Build history of the part. All positions in model axes, mm. A direction names the side the tool comes from. Round coordinates to 2 decimals unless told otherwise and drop trailing zeros. Use one line per item in the form item = value. Start each with the question number.
```python
from build123d import *

# Parameters (mm, degrees)
F0_R     = 37
F1_DEPTH = 2
F2_R     = 38
F3_DEPTH = 3
F4_R     = 37
F5_DEPTH = 2
F6_R     = 38
F7_DEPTH = 3
F8_R     = 37
F9_DEPTH = 2


# Not quite as in the source:
# - a fillet or chamfer that OpenCascade refuses, or shapes differently, is made with other operations: its cross-section is extruded or revolved along the edge and cut away or added


with BuildPart() as f1:
    # F0 (on Top) → F1 (new body)
    with BuildSketch(Plane.XY):
        Circle(F0_R)
    extrude(amount=F1_DEPTH)

    # F2 (on face) → F3 (join)
    with BuildSketch(Plane.XY.offset(2)):
        Circle(F2_R)
    extrude(amount=F3_DEPTH)

    # F4 (on face) → F5 (join)
    with BuildSketch(Plane.XY.offset(5)):
        Circle(F4_R)
    extrude(amount=F5_DEPTH)

    # F6 (on face) → F7 (join)
    with BuildSketch(Plane.XY.offset(7)):
        Circle(F6_R)
    extrude(amount=F7_DEPTH)

    # F8 (on face) → F9 (join)
    with BuildSketch(Plane.XY.offset(10)):
        Circle(F8_R)
    extrude(amount=F9_DEPTH)

    # F10: fillet of radius 1.6 on 4 edges, made by hand

    # F10_s1 → F10_t2 (revolve, cut)
    with BuildSketch(Plane.XZ):
        with BuildLine():
            ThreePointArc((38, 8.4832396974), (37.7266499161, 7.5888125064), (37, 7))
            Line((37, 7), (38, 7))
            Line((38, 7), (38, 8.4832396974))
        make_face()
    revolve(axis=Axis((0, 0, 7), (0, 0, 1)), mode=Mode.SUBTRACT)

    # F10_s3 → F10_t4 (revolve, cut)
    with BuildSketch(Plane.XZ):
        with BuildLine():
            ThreePointArc((38, 3.4832396974), (37.7266499161, 2.5888125064), (37, 2))
            Line((37, 2), (38, 2))
            Line((38, 2), (38, 3.4832396974))
        make_face()
    revolve(axis=Axis((0, 0, 2), (0, 0, 1)), mode=Mode.SUBTRACT)

    # F10_s5 → F10_t6 (revolve, cut)
    with BuildSketch(Plane.XZ):
        with BuildLine():
            ThreePointArc((38, 8.5167603026), (37.7266499161, 9.4111874936), (37, 10))
            Line((37, 10), (38, 10))
            Line((38, 10), (38, 8.5167603026))
        make_face()
    revolve(axis=Axis((0, 0, 10), (0, 0, 1)), mode=Mode.SUBTRACT)

    # F10_s7 → F10_t8 (revolve, cut)
    with BuildSketch(Plane.XZ):
        with BuildLine():
            ThreePointArc((37, 5), (37.7266499161, 4.4111874936), (38, 3.5167603026))
            Line((38, 3.5167603026), (38, 5))
            Line((38, 5), (37, 5))
        make_face()
    revolve(axis=Axis((0, 0, 5), (0, 0, 1)), mode=Mode.SUBTRACT)


solid = f1.part
```
Q1. Drop flat-ended pins along their axis: P1, Ø10, axis at x = 23, y = -30, coming from the +Z side; P2, Ø2, axis at x = -25.5, z = 9, coming from the -Y side; P3, Ø4, axis at y = 9, z = 7.5, coming from the +X side; P4, Ø1.5, axis at y = -6, z = 10.5, coming from the -X side. Give the stop position or say it passes through.
Q2. Wall check: probe 1 along X at (y, z) = (-1, 8.5); probe 2 along X at (y, z) = (34, 4.5); probe 3 along Y at (x, z) = (-7, 9.5). Give the ranges that are in metal, low to high.
Q3. Tool access for faces 1 (the face through (-8.02, -36.12, 10.99)), 2 (the face through (-8.02, -36.12, 0.99)), 3 (the face through (-1, 1, 12)), 4 (the face through (-1, 1, 0)), 5 (the face through (-8.02, -36.12, 5.99)): list every direction of +Z, -Z, +X, -X, +Y, -Y with a clear straight run to the whole face (end or side of a thin tool).
Filled in:
q1.P1 = 12
q1.P2 = -29
q1.P3 = 37.31
q1.P4 = -36.94
q2.probe_1 = -37.99 to 37.99
q2.probe_2 = -16.2 to 16.2
q2.probe_3 = -37.01 to 37.01
q3.face_1 = +Z
q3.face_2 = -Z
q3.face_3 = +Z, +X, -X, +Y, -Y
q3.face_4 = -Z, +X, -X, +Y, -Y
q3.face_5 = none
